from build123d import *

# Parameters (mm, degrees)
SKETCH1_W            = 88.03
SKETCH1_H            = 88.03
SKETCH1_W_2          = 78.03
SKETCH1_H_2          = 78.03
BOSS_EXTRUDE1_DEPTH  = 20
SKETCH2_W            = 16
SKETCH2_H            = 15
CUT_EXTRUDE1_DEPTH   = 20
SKETCH5_W            = 12
SKETCH5_H            = 10
BOSS_EXTRUDE2_DEPTH  = 20
SKETCH3_W            = 0.15
SKETCH3_H            = 15
CUT_EXTRUDE2_DEPTH   = 73.490968058
CUT_EXTRUDE3_DEPTH   = 2.5
SKETCH7_R            = 1.55
CUT_EXTRUDE4_DEPTH   = 77.283159675
SKETCH8_W            = 16
SKETCH8_H            = 5
BOSS_EXTRUDE3_DEPTH  = 20
CUT_EXTRUDE5_DEPTH   = 117.669109558
FILLET8_R            = 2
FILLET8_OF_MIRROR9_R = 2
CHAMFER1_SIZE        = 4
SKETCH10_W           = 15
SKETCH10_H           = 16
CUT_EXTRUDE6_DEPTH   = 15
FILLET7_R            = 1.5
CHAMFER2_SIZE        = 1
CHAMFER3_SIZE        = 0.5


with BuildPart() as part:
    # Sketch1 → Boss-Extrude1 (new body)
    with BuildSketch(Plane.XY):
        Rectangle(SKETCH1_W, SKETCH1_H)
        Rectangle(SKETCH1_W_2, SKETCH1_H_2, mode=Mode.SUBTRACT)
    extrude(amount=BOSS_EXTRUDE1_DEPTH)

    # Sketch2 → Cut-Extrude1 (cut)
    with BuildSketch(Plane(origin=(44.015, 0, 0), x_dir=(0, 0, -1), z_dir=(1, 0, 0))):
        with Locations((-8, -31.515)):
            Rectangle(SKETCH2_W, SKETCH2_H)
    extrude(amount=-CUT_EXTRUDE1_DEPTH, mode=Mode.SUBTRACT)

    # Sketch5 → Boss-Extrude2 (add)
    with BuildSketch(Plane(origin=(0, 0, 0), x_dir=(-1, 0, 0), z_dir=(0, 0, -1))):
        with Locations((0, -49.015)):
            Rectangle(SKETCH5_W, SKETCH5_H)
    extrude(amount=-BOSS_EXTRUDE2_DEPTH)

    # Sketch3 → Cut-Extrude2 (cut, through all)
    with BuildSketch(Plane(origin=(0, 0, 0), x_dir=(-1, 0, 0), z_dir=(0, 0, -1))):
        with Locations((0, -46.515)):
            Rectangle(SKETCH3_W, SKETCH3_H)
    extrude(amount=-CUT_EXTRUDE2_DEPTH, mode=Mode.SUBTRACT)

    # Sketch6 → Cut-Extrude3 (cut)
    with BuildSketch(Plane.ZY.offset(6)):
        Polygon((8.5, -47.42728676), (5.75, -45.839573519), (3, -47.42728676), (3, -50.60271324), (5.75, -52.190426481), (8.5, -50.60271324), align=None)
        Polygon((17, -47.42728676), (14.25, -45.839573519), (11.5, -47.42728676), (11.5, -50.60271324), (14.25, -52.190426481), (17, -50.60271324), align=None)
    cut_extrude3 = extrude(amount=-CUT_EXTRUDE3_DEPTH, mode=Mode.SUBTRACT)

    # Sketch7 → Cut-Extrude4 (cut, symmetric)
    with BuildSketch(Plane.ZY.offset(6)):
        with Locations(Location((5.75, -49.015, 0), (0, 0, 270))):
            Circle(SKETCH7_R)
        with Locations(Location((14.25, -49.015, 0), (0, 0, 270))):
            Circle(SKETCH7_R)
    cut_extrude4 = extrude(amount=CUT_EXTRUDE4_DEPTH, both=True, mode=Mode.SUBTRACT)

    # Sketch8 → Boss-Extrude3 (add)
    with BuildSketch(Plane(origin=(0, 0, 0), x_dir=(-1, 0, 0), z_dir=(0, 0, -1))):
        with Locations((-52.015, 41.515)):
            Rectangle(SKETCH8_W, SKETCH8_H)
    boss_extrude3 = extrude(amount=-BOSS_EXTRUDE3_DEPTH)

    # Sketch9 → Cut-Extrude5 (cut, through all)
    with BuildSketch(Plane(origin=(0, 44.015, 0), x_dir=(1, 0, 0), z_dir=(0, 1, 0))):
        with BuildLine():
            Line((52.015, -14.4), (56.015, -14.4))
            ThreePointArc((56.015, -14.4), (57.615, -16), (56.015, -17.6))
            Line((56.015, -17.6), (52.015, -17.6))
            ThreePointArc((52.015, -17.6), (50.415, -16), (52.015, -14.4))
        make_face()
        with BuildLine():
            Line((52.015, -2.4), (56.015, -2.4))
            ThreePointArc((56.015, -2.4), (57.615, -4), (56.015, -5.6))
            Line((56.015, -5.6), (52.015, -5.6))
            ThreePointArc((52.015, -5.6), (50.415, -4), (52.015, -2.4))
        make_face()
    cut_extrude5 = extrude(amount=-CUT_EXTRUDE5_DEPTH, mode=Mode.SUBTRACT)

    # Fillet8
    fillet8_edges = [part.edges().sort_by_distance(p)[0] for p in [
        (60.015, 41.515, 0),
        (60.015, 41.515, 20),
    ]]
    fillet(fillet8_edges, radius=FILLET8_R)

    # Mirror9: Cut-Extrude3, Cut-Extrude4, Boss-Extrude3, Cut-Extrude5 across plane
    add(cut_extrude3.mirror(Plane(origin=(0, 0, 0), x_dir=(0, 0, 1), z_dir=(1, 0, 0))), mode=Mode.SUBTRACT)
    add(cut_extrude4.mirror(Plane(origin=(0, 0, 0), x_dir=(0, 0, 1), z_dir=(1, 0, 0))), mode=Mode.SUBTRACT)
    add(boss_extrude3.mirror(Plane(origin=(0, 0, 0), x_dir=(0, 0, 1), z_dir=(1, 0, 0))))
    add(cut_extrude5.mirror(Plane(origin=(0, 0, 0), x_dir=(0, 0, 1), z_dir=(1, 0, 0))), mode=Mode.SUBTRACT)

    # Fillet8 of Mirror9
    fillet8_of_mirror9_edges = [part.edges().sort_by_distance(p)[0] for p in [
        (-60.015, 41.515, 0),
        (-60.015, 41.515, 20),
    ]]
    fillet(fillet8_of_mirror9_edges, radius=FILLET8_OF_MIRROR9_R)

    # Chamfer1
    chamfer1_edges = [part.edges().sort_by_distance(p)[0] for p in [
        (44.015, 39.015, 10),
        (-44.015, 39.015, 10),
    ]]
    chamfer(chamfer1_edges, length=CHAMFER1_SIZE)

    # Sketch10 → Cut-Extrude6 (cut)
    with BuildSketch(Plane.XZ.offset(44.015)):
        with Locations((-31.515, 8)):
            Rectangle(SKETCH10_W, SKETCH10_H)
    extrude(amount=-CUT_EXTRUDE6_DEPTH, mode=Mode.SUBTRACT)

    # Fillet7
    fillet7_edges = [part.edges().sort_by_distance(p)[0] for p in [
        (-39.015, -41.515, 16),
        (-24.015, -41.515, 16),
        (41.515, -39.015, 16),
        (41.515, -24.015, 16),
    ]]
    fillet(fillet7_edges, radius=FILLET7_R)

    # Chamfer2
    chamfer2_edges = [part.edges().sort_by_distance(p)[0] for p in [
        (0, 39.015, 0),
        (-39.015, -2.5, 0),
        (39.015, 0, 20),
        (0, 39.015, 20),
        (-39.015, 0, 20),
        (-19.545, -39.015, 20),
        (39.015, 7.5, 0),
        (-12.045, -39.015, 0),
        (-6, -54.015, 10),
        (-6, -44.015, 10),
        (6, -44.015, 10),
        (6, -54.015, 10),
        (22.045, -39.015, 0),
        (19.545, -39.015, 20),
        (0.075, -54.015, 10),
        (0.075, -39.015, 10),
        (-0.075, -39.015, 10),
        (-0.075, -54.015, 10),
    ]]
    chamfer(chamfer2_edges, length=CHAMFER2_SIZE)

    # Chamfer3
    chamfer3_edges = [part.edges().sort_by_distance(p)[0] for p in [
        (54.015, 39.015, 5.6),
        (57.615, 39.015, 4),
        (54.015, 39.015, 2.4),
        (50.415, 39.015, 4),
        (54.015, 39.015, 17.6),
        (57.615, 39.015, 16),
        (54.015, 39.015, 14.4),
        (50.415, 39.015, 16),
        (50.415, 44.015, 16),
        (54.015, 44.015, 17.6),
        (57.615, 44.015, 16),
        (54.015, 44.015, 14.4),
        (50.415, 44.015, 4),
        (54.015, 44.015, 5.6),
        (57.615, 44.015, 4),
        (54.015, 44.015, 2.4),
        (-54.015, 39.015, 2.4),
        (-57.615, 39.015, 4),
        (-54.015, 39.015, 5.6),
        (-50.415, 39.015, 4),
        (-54.015, 39.015, 14.4),
        (-57.615, 39.015, 16),
        (-54.015, 39.015, 17.6),
        (-50.415, 39.015, 16),
        (-50.415, 44.015, 16),
        (-54.015, 44.015, 17.6),
        (-57.615, 44.015, 16),
        (-54.015, 44.015, 14.4),
        (-50.415, 44.015, 4),
        (-54.015, 44.015, 5.6),
        (-57.615, 44.015, 4),
        (-54.015, 44.015, 2.4),
    ]]
    chamfer(chamfer3_edges, length=CHAMFER3_SIZE)


solid = part.part
For this review, take the finished solid that the model builds, in its own axes (mm). A direction names the side the tool comes from. Give positions to 0.01 mm unless a question says otherwise; leave off trailing zeros. Loops run counter-clockwise (first coordinate to the right, second up) from the corner with the lowest first, then second, coordinate; pieces in that order, holes last. Notation, with made-up numbers: M -26.5,32 L 11.5,32 A26 ccw 11.5,58 Z; hole C 43.25,67.5 d10. An arc over 180 degrees is marked long. Answer as a JSON object with one key per item and string values. Group by question number.
Q1. Insertion check: P1, Ø10, axis at x = -17.5, z = 3, coming from the -Y side (3 decimals); P2, Ø10.5, axis at y = -48, z = 13, coming from the -X side (3 decimals); P3, Ø4, axis at y = -49.015, z = 5.75, coming from the +X side. Each pin has a flat end and moves straight along its axis. Give the tip position at first contact, or say it passes through.
Q2. Tool access review of faces 4 (the flat face through (-12, -39.015, 10)), 5 (the flat face through (-5, -49, 17)), 6 (the flat face through (54, 39.015, 10)): name each direction out of +Z, -Z, +X, -X, +Y, -Y from which nothing blocks a thin tool from reaching the whole face with its end or side.
Q3. For probe 1 along X at (y, z) = (-20, 2) (3 decimals); probe 2 along Z at (x, y) = (4, -46.5), list the stretches that pass through material, from the lowest coordinate up. Write a range as [from, to].
Q4. Add section B-B on x = 33.5. Give the boundary of the cut face in (y, z) (3 decimals), and give its area (3 significant figures).
Q5. Add section A-A on y = -32. Give the boundary of the cut face in (x, z) (3 decimals).
Q6. Mouldability with a two-part tool opening along Z and no side actions: class faces 1 (the cylindrical face through (-57.615, 41.543, 15.965)), 2 (the flat face through (3, -54.015, 10)), 3 (the flat face through (-5, 43, 0)) as +Z half, -Z half, draft (parallel to the pull), parting line (faces both ways), or undercut.
Checked values:
{
 "1": {"P1": "y = -44.015", "P2": "x = -44.015", "P3": "x = 3.5"},
 "2": {"face 4": "+Z, -Z", "face 5": "-X", "face 6": "+Z, -Z, +X, -Y"},
 "3": {"probe 1": "[-44.015, -39.015], [39.015, 44.015]", "probe 2": "[0, 4.61], [6.89, 13.11], [15.39, 20]"},
 "4": {"outline": "M -44.015,0 L -40.015,0 L -39.015,1 L -39.015,19 L -40.015,20 L -44.015,20 Z; M 39.015,1 L 40.015,0 L 44.015,0 L 44.015,20 L 40.015,20 L 39.015,19 Z", "area": "198 mm²"},
 "5": {"outline": "M -44.015,0 L -40.015,0 L -39.015,1 L -39.015,19 L -40.015,20 L -44.015,20 Z; M 39.015,16 L 44.015,16 L 44.015,20 L 40.015,20 L 39.015,19 Z"},
 "6": {"face 1": "undercut", "face 2": "draft", "face 3": "-Z half"}
}
